Autodesk Inventor part; units mm, degrees
ref_plane "YZ Plane" through (0, 0, 0) normal (1, 0, 0) x (0, 1, 0)
ref_plane "XZ Plane" through (0, 0, 0) normal (0, 1, 0) x (-1, 0, 0)
ref_plane "XY Plane" through (0, 0, 0) normal (0, 0, 1) x (1, 0, 0)
sketch "Skizze1" plane through (0, 0, 0) normal (0, 1, 0) x (-1, 0, 0)
  line L0 (0, 0) -> (-132.5, 0)
  line L1 (-132.5, 0) -> (-132.5, 122.5)
  line L2 (-132.5, 122.5) -> (0, 122.5)
  line L3 (0, 122.5) -> (0, 0)
  dimension "d0" = 132.5
  dimension "d1" = 122.5
extrude "Extrusion1" add sketch "Skizze1" along normal blind 30
sketch "Skizze2" plane through (0, 30, 0) normal (0, 1, 0) x (1, 0, 0)
  line L0 (0, 0) -> (11.25, 0)
  line L1 (11.25, 0) -> (11.25, -6.25)
  line L2 (11.25, -6.25) -> (121.25, -6.25)
  line L3 (121.25, -6.25) -> (121.25, -116.25)
  line L4 (121.25, -116.25) -> (11.25, -116.25)
  line L5 (11.25, -116.25) -> (11.25, -6.25)
  dimension "d4" = 11.25
  dimension "d5" = 6.25
  dimension "d6" = 110
  dimension "d7" = 110
extrude "Extrusion2" cut sketch "Skizze2" against normal blind 25
sketch "Skizze3" plane through (0, 0, 0) normal (-1, 0, 0) x (0, 0, 1)
  line L0 (0, 29.9998) -> (20, 29.9998)
  line L1 (20, 29.9998) -> (20, 19.9998)
  line L2 (20, 19.9998) -> (0, 19.9998)
  line L3 (0, 19.9998) -> (0, 29.9998)
  line L4 (122.5002, 29.9998) -> (102.5002, 29.9998)
  line L5 (102.5002, 29.9998) -> (102.5002, 19.9998)
  line L6 (102.5002, 19.9998) -> (122.5002, 19.9998)
  line L7 (122.5002, 19.9998) -> (122.5002, 29.9998)
  point P0 (0, 0)
  dimension "d10" = 20
  dimension "d11" = 10
  dimension "d12" = 20
  dimension "d13" = 10
extrude "Extrusion3" add sketch "Skizze3" along normal blind 20
sketch "Skizze4" plane through (132.5, 0, 122.5) normal (1, 0, 0) x (0, 0, -1)
  line L0 (0.0001, 29.9997) -> (20.0001, 29.9997)
  line L1 (20.0001, 29.9997) -> (20.0001, 19.9997)
  line L2 (20.0001, 19.9997) -> (0.0001, 19.9997)
  line L3 (0.0001, 19.9997) -> (0.0001, 29.9997)
  line L4 (122.5, 29.9997) -> (102.5, 29.9997)
  line L5 (102.5, 29.9997) -> (102.5, 19.9997)
  line L6 (102.5, 19.9997) -> (122.5, 19.9997)
  line L7 (122.5, 19.9997) -> (122.5, 29.9997)
  point P0 (122.5, 0)
  dimension "d16" = 20
  dimension "d17" = 10
  dimension "d18" = 20
  dimension "d19" = 10
extrude "Extrusion4" add sketch "Skizze4" along normal blind 20
sketch "Skizze5" plane through (0, 29.9998, 122.5) normal (0, 1, 0) x (1, 0, 0)
  line L0 (0, 19.9998) -> (-20, 19.9998)
  line L1 (-20, -0.0002) -> (-20, 19.9998)
  point P0 (0, 122.5)
  point P1 (-10, 9.9998)
  dimension "d22" = 10
  dimension "d23" = 10
hole "Bohrung1" at (-10, 29.9998, 112.5002) direction (0, -1, 0) diameter 5 end through all
sketch "Skizze6" plane through (0, 29.9998, 20) normal (0, 1, 0) x (1, 0, 0)
  line L0 (0, 20) -> (-20, 20)
  line L1 (-20, 0) -> (-20, 20)
  point P0 (-10, 10)
  dimension "d31" = 10
  dimension "d32" = 10
hole "Bohrung2" at (-10, 29.9998, 10) direction (0, -1, 0) diameter 5 end through all
sketch "Skizze7" plane through (132.5, 29.9997, 122.4999) normal (0, 1, 0) x (1, 0, 0)
  line L0 (0, 20) -> (20, 20)
  line L1 (20, 20) -> (20, 0)
  point P0 (-132.5, 122.4999)
  point P1 (10, 10)
  dimension "d40" = 10
  dimension "d41" = 10
hole "Bohrung3" at (142.5, 29.9997, 112.4999) direction (0, -1, 0) diameter 5 end through all
sketch "Skizze8" plane through (132.5, 29.9997, 20) normal (0, 1, 0) x (1, 0, 0)
  line L0 (0, 20) -> (20, 20)
  line L1 (20, 20) -> (20, 0)
  point P0 (-132.5, 20)
  point P1 (10, 10)
  dimension "d49" = 10
  dimension "d50" = 10
hole "Bohrung4" at (142.5, 29.9997, 10) direction (0, -1, 0) diameter 5 end through all
thread "Gewinde1"
thread "Gewinde2"
thread "Gewinde3"
thread "Gewinde4"
properties part number "Oberteil"
Read the model definition and answer for the solid it produces. Units are mm, in the model's axes. A direction names the side the tool comes from. Give positions to 0.01 mm unless a question says otherwise; leave off trailing zeros. Loops run counter-clockwise (first coordinate to the right, second up) from the corner with the lowest first, then second, coordinate; pieces in that order, holes last.
Item 1: The mould has two halves that part along Z. Classify faces 6 (the cylindrical face through (140.39, 24.93, 113.84)), 7 (the flat face through (65, 15, 0)), 8 (the flat face through (-8, 20, 12)), 9 (the flat face through (-10, 25, 122.5)): released by +Z, released by -Z, zero draft, split by the parting line, or undercut.
Item 2: The part is cut by section A-A (y = 21.75). Give the number of separate pieces and of enclosed holes in the cut face, and give its area (3 significant figures).
Item 3: Find the intervals of material crossed by line 1 along Z through (x, y) = (-10, 24); line 2 along Z through (x, y) = (61.5, 14.5); line 3 along X through (y, z) = (17, 15.5), in increasing order.
Item 4: For faces 1 (the flat face through (142, 25, 20)), 2 (the flat face through (-10, 25, 20)), 3 (the flat face through (-20, 25, 10)), 4 (the flat face through (-8, 20, 115)), 5 (the flat face through (121.25, 18, 60)), determine the directions among +Z, -Z, +X, -X, +Y, -Y from which every point of the face is accessible in a straight line to the end or side of a thin tool.
Item 5: Each of these flat-tipped pins is pushed along its axis until it touches: pin 1 Ø5 at (y, z) = (24.5, 66) entering from +X; pin 2 Ø6 at (x, z) = (-8.5, 116.5) entering from -Y; pin 3 Ø6 at (x, z) = (107.5, 17) entering from +Y. Where does it stop, or does it pass through?
Item 6: The part is cut by section D-D (y = 13.5). Write down the section's boundary in (x, z), and give its area (3 significant figures).
Item 7: The part is cut by section C-C (x = -10). Write down the section's boundary in (y, z).
Taken from the geometry:
1. face 6: undercut
1. face 7: released by -Z
1. face 8: zero draft
1. face 9: released by +Z
2. separate pieces: 1
2. enclosed holes: 5
2. area: 5,650 mm2
3. line 1: z = 0 to 7.5, 12.5 to 20, 102.5 to 110, 115 to 122.5
3. line 2: z = 0 to 6.25, 116.25 to 122.5
3. line 3: x = 0 to 11.25, 121.25 to 132.5
4. face 1: +X, +Y, -Y
4. face 2: -X, +Y, -Y
4. face 3: +Z, -Z, -X, +Y, -Y
4. face 4: +Z, -Z, -X, -Y
4. face 5: +Y
5. pin 1: stops at x = 132.5
5. pin 2: stops at y = 20
5. pin 3: stops at y = 5
6. outline: (0, 0) - (132.5, 0) - (132.5, 122.5) - (0, 122.5) - close; hole (11.25, 6.25) - (121.25, 6.25) - (121.25, 116.25) - (11.25, 116.25) - close
6. area: 4,130 mm2
7. outline: (20, 0) - (30, 0) - (30, 7.5) - (20, 7.5) - close; (20, 12.5) - (30, 12.5) - (30, 20) - (20, 20) - close; (20, 102.5) - (30, 102.5) - (30, 110) - (20, 110) - close; (20, 115) - (30, 115) - (30, 122.5) - (20, 122.5) - close
